Part model, mm, in its own coordinate system. Face numbers are marked on the shaded views. A direction names the side the tool comes from. Coordinates: 2 decimals unless noted, no trailing zeros. Loops run counter-clockwise (first coordinate to the right, second up) from the corner with the lowest first, then second, coordinate; pieces in that order, holes last. Notation, with made-up numbers: M -34,-31.75 L 15,-31.75 A15 ccw 15,-15.75 Z; hole C -24.75,-31.5 d1. An arc over 180 degrees is marked long. Use CSV: the item, a comma, the result in double quotes. Start each with the question number.
from build123d import *

# Parameters (mm, degrees)
SKETCH_1_R          = 15
EXTRUDE_1_DEPTH     = 35
SKETCH_2_R          = 1.4
CUT_EXTRUDE_1_DEPTH = 41.926763859
SKETCH_4_W          = 10.3
SKETCH_4_H          = 8.64
SKETCH_4_W_2        = 6.34
SKETCH_4_H_2        = 6.34
EXTRUDE_2_DEPTH     = 8
SKETCH_5_W          = 10.3
SKETCH_5_H          = 20.03
CUT_EXTRUDE_2_DEPTH = 5
CUT_EXTRUDE_3_DEPTH = 50.751390935
CUT_EXTRUDE_4_DEPTH = 37.742346142
SKETCH_8_W          = 2.3
SKETCH_8_H          = 6.34
EXTRUDE_3_DEPTH     = 1.6
SKETCH_10_W         = 2.02
SKETCH_10_H         = 3
SKETCH_11_W         = 6.34
SKETCH_11_H         = 6.34
CUT_EXTRUDE_5_DEPTH = 6.5
SKETCH_12_W         = 2.02
SKETCH_12_H         = 3
CUT_EXTRUDE_7_DEPTH = 5
SKETCH_16_R         = 3.19
CUT_EXTRUDE_8_DEPTH = 1.2
CUT_EXTRUDE_9_DEPTH = 41.926763859
CHAMFER_1_SIZE      = 1.1
CHAMFER_2_SIZE      = 1


with BuildPart() as part:
    # 草图1 → 凸台-拉伸1 (new body)
    with BuildSketch(Plane(origin=(0, 0, 0), x_dir=(1, 0, 0), z_dir=(0, 1, 0))):
        with Locations(Location((0, 0, 0), (0, 0, 270))):
            Circle(SKETCH_1_R)
    extrude(amount=EXTRUDE_1_DEPTH)

    # 草图2 → 切除-拉伸1 (cut, through all)
    with BuildSketch(Plane(origin=(0, 35, 0), x_dir=(1, 0, 0), z_dir=(0, 1, 0))):
        with Locations(Location((9, 0, 0), (0, 0, 270))):
            Circle(SKETCH_2_R)
        with Locations(Location((-9, 0, 0), (0, 0, 90))):
            Circle(SKETCH_2_R)
    extrude(amount=-CUT_EXTRUDE_1_DEPTH, mode=Mode.SUBTRACT)

    # 草图4 → 凸台-拉伸2 (add)
    with BuildSketch(Plane(origin=(0, 35, 0), x_dir=(1, 0, 0), z_dir=(0, 1, 0))):
        with Locations((0, -9.35)):
            Rectangle(SKETCH_4_W, SKETCH_4_H)
        with Locations((0, -9)):
            Rectangle(SKETCH_4_W_2, SKETCH_4_H_2, mode=Mode.SUBTRACT)
    extrude(amount=EXTRUDE_2_DEPTH)

    # 草图5 → 切除-拉伸2 (cut)
    with BuildSketch(Plane(origin=(0, 35, 0), x_dir=(1, 0, 0), z_dir=(0, 1, 0))):
        with Locations((0, 4.985)):
            Rectangle(SKETCH_5_W, SKETCH_5_H)
    extrude(amount=-CUT_EXTRUDE_2_DEPTH, mode=Mode.SUBTRACT)

    # 草图6 → 切除-拉伸3 (cut, through all)
    with BuildSketch(Plane(origin=(0, 0, 5.03), x_dir=(-1, 0, 0), z_dir=(0, 0, -1))):
        Polygon((-6.15, 32.5), (-5.15, 33.75), (-5.15, 31.25), align=None)
        Polygon((6.15, 32.5), (5.15, 33.75), (5.15, 31.25), align=None)
    extrude(amount=CUT_EXTRUDE_3_DEPTH, mode=Mode.SUBTRACT)

    # 草图7 → 切除-拉伸4 (cut, through all)
    with BuildSketch(Plane(origin=(0, 30, 0), x_dir=(1, 0, 0), z_dir=(0, 1, 0))):
        with BuildLine():
            Line((-5.15, 14.088204286), (-5.15, 4.97))
            Line((-5.15, 4.97), (5.15, 4.97))
            Line((5.15, 4.97), (5.15, 14.088204286))
            ThreePointArc((5.15, 14.088204286), (0, 15), (-5.15, 14.088204286))
        make_face()
    extrude(amount=-CUT_EXTRUDE_4_DEPTH, mode=Mode.SUBTRACT)

    # 草图8 → 凸台-拉伸3 (add)
    with BuildSketch(Plane(origin=(0, 35, 0), x_dir=(1, 0, 0), z_dir=(0, 1, 0))):
        with Locations((0, -9)):
            Rectangle(SKETCH_8_W, SKETCH_8_H)
    extrude(amount=EXTRUDE_3_DEPTH)

    # 切除-扫描1: sweep along a path in 草图9
    with BuildLine(Plane(origin=(0, 0, 0), x_dir=(0, 0, -1), z_dir=(1, 0, 0))) as sweep_1_path:
        Line((-9, 35), (-9, 27.97))
        Line((-9, 27.97), (-3.03, 22))
        Line((-3.03, 22), (4.97, 22))
    # 草图10 → 切除-扫描1 (sweep, cut)
    with BuildSketch(Plane(origin=(0, 35, 0), x_dir=(1, 0, 0), z_dir=(0, 1, 0))):
        with Locations((2.16, -9)):
            Rectangle(SKETCH_10_W, SKETCH_10_H)
        with Locations((-2.16, -9)):
            Rectangle(SKETCH_10_W, SKETCH_10_H)
    sweep(path=sweep_1_path.line, transition=Transition.RIGHT, mode=Mode.SUBTRACT)

    # 草图11 → 切除-拉伸5 (cut)
    with BuildSketch(Plane.XZ):
        with Locations((0, 9)):
            Rectangle(SKETCH_11_W, SKETCH_11_H)
    extrude(amount=-CUT_EXTRUDE_5_DEPTH, mode=Mode.SUBTRACT)

    # 切除-扫描2: sweep along a path in 草图13
    with BuildLine(Plane(origin=(0, 0, 0), x_dir=(0, 0, -1), z_dir=(1, 0, 0))) as sweep_2_path:
        Line((-9, 6.5), (-9, 13.5))
        Line((-9, 13.5), (-4.5, 18))
        Line((-4.5, 18), (4.97, 18))
    # 草图12 → 切除-扫描2 (sweep, cut)
    with BuildSketch(Plane.XZ.offset(-6.5)):
        with Locations((-2.16, 9)):
            Rectangle(SKETCH_12_W, SKETCH_12_H)
        with Locations((2.16, 9)):
            Rectangle(SKETCH_12_W, SKETCH_12_H)
    sweep(path=sweep_2_path.line, transition=Transition.RIGHT, mode=Mode.SUBTRACT)

    # 草图15 → 切除-拉伸7 (cut)
    with BuildSketch(Plane(origin=(0, 35, 0), x_dir=(1, 0, 0), z_dir=(0, 1, 0))):
        Polygon((9, 2.615396719), (6.735, 1.30769836), (6.735, -1.30769836), (9, -2.615396719), (11.265, -1.30769836), (11.265, 1.30769836), align=None)
        Polygon((-11.265, -1.30769836), (-11.265, 1.30769836), (-9, 2.615396719), (-6.735, 1.30769836), (-6.735, -1.30769836), (-9, -2.615396719), align=None)
    cut_extrude_7 = extrude(amount=-CUT_EXTRUDE_7_DEPTH, mode=Mode.SUBTRACT)

    # 草图16 → 切除-拉伸8 (cut)
    with BuildSketch(Plane(origin=(0, 35, 0), x_dir=(1, 0, 0), z_dir=(0, 1, 0))):
        with Locations(Location((9, 0, 0), (0, 0, 270))):
            Circle(SKETCH_16_R)
        with Locations(Location((-9, 0, 0), (0, 0, 90))):
            Circle(SKETCH_16_R)
    cut_extrude_8 = extrude(amount=-CUT_EXTRUDE_8_DEPTH, mode=Mode.SUBTRACT)

    # 镜向1: 切除-拉伸7, 切除-拉伸8 across plane
    add(cut_extrude_7.mirror(Plane.ZX.offset(17.5)), mode=Mode.SUBTRACT)
    add(cut_extrude_8.mirror(Plane.ZX.offset(17.5)), mode=Mode.SUBTRACT)

    # 草图17 → 切除-拉伸9 (cut, through all)
    with BuildSketch(Plane(origin=(0, 35, 0), x_dir=(1, 0, 0), z_dir=(0, 1, 0))):
        with BuildLine():
            Line((14.5, 3.840572874), (14.5, -3.840572874))
            ThreePointArc((14.5, -3.840572874), (15, 0), (14.5, 3.840572874))
        make_face()
        with BuildLine():
            Line((-14.5, 3.840572874), (-14.5, -3.840572874))
            ThreePointArc((-14.5, -3.840572874), (-15, 0), (-14.5, 3.840572874))
        make_face()
    extrude(amount=-CUT_EXTRUDE_9_DEPTH, mode=Mode.SUBTRACT)

    # 倒角1
    # the kernel refuses this chamfer: 1.1 mm, written as the material it adds along each edge
    with BuildSketch(Plane(origin=(-3.17, 19.5, 7.95017163), x_dir=(-0.027495876610586133, -0.9996219169112966, 0), z_dir=(0, 0, -1))) as chamfer_1_piece_1:
        Polygon((CHAMFER_1_SIZE * 0.999621916911, -CHAMFER_1_SIZE * 0.0274958766106), (-CHAMFER_1_SIZE * 0.0274958766106, -CHAMFER_1_SIZE * 0.999621916911), (0, 0), align=None)
    extrude(amount=12.92017163)
    with BuildSketch(Plane(origin=(-1.15, 19.5, 7.95017163), x_dir=(0.02749587661058633, -0.9996219169112966, 0), z_dir=(0, 0, -1)), Plane(origin=(3.17, 19.5, 7.95017163), x_dir=(0.027495876610586525, -0.9996219169112966, 0), z_dir=(0, 0, -1)), Plane(origin=(1.15, 19.5, 7.95017163), x_dir=(0.9996219169112966, 0.02749587661058971, 0), z_dir=(0, 0, -1))) as chamfer_1_piece_2:
        Polygon((CHAMFER_1_SIZE * 0.999621916911, CHAMFER_1_SIZE * 0.0274958766106), (-CHAMFER_1_SIZE * 0.0274958766106, CHAMFER_1_SIZE * 0.999621916911), (0, 0), align=None)
    extrude(amount=12.92017163)

    # 倒角2
    chamfer_2_edges = [part.edges().sort_by_distance(p)[0] for p in [
        (3.17, 23.5, -1.280660172),
        (1.15, 23.5, -1.280660172),
        (-1.15, 23.5, -1.280660172),
        (-3.17, 23.5, -1.280660172),
    ]]
    chamfer(chamfer_2_edges, length=CHAMFER_2_SIZE)


solid = part.part
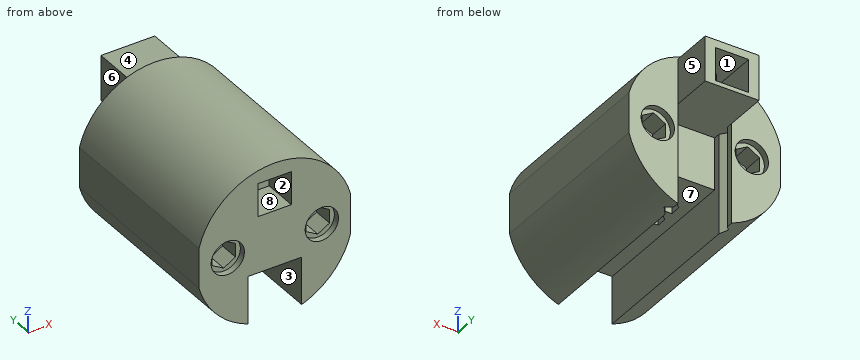
1. Slice it at C-C, the plane x = 9.5. List the corners of the cut face in (y, z), and give its area (3 significant figures).
2. Two-plate mould, pull along Z, no slides. Class the marked faces 1, 2, 3 and 4: pulls with the +Z half, pulls with the -Z half, needs draft (parallel to the pull), parting line crosses it, or undercut.
3. Slice it at A-A, the plane y = 34.5. List the corners of the cut face in (x, z), and give its area (3 significant figures).
4. Slice it at B-B, the plane z = -11.25. List the corners of the cut face in (x, y).
5. Pin check, flat tips, straight feed: pin 1 (2 mm diameter, centred on x = -2, y = 27, fed in from +Z); pin 2 (2 mm diameter, centred on y = 36.5, z = 12, fed in from -X); pin 3 (1.2 mm diameter, centred on x = 0, z = 9.5, fed in from +Y). Stop position of each tip, or through.
6. Slice it at D-D, the plane z = 0. State how many separate pieces and enclosed holes the cut face has, and give its area (3 significant figures).
7. Wall check: probe 1 along X at (y, z) = (0.7, 0); probe 2 along X at (y, z) = (16, 0); probe 3 along X at (y, z) = (34.5, 0). Give the ranges that are in metal, low to high.
8. Tool access for the marked faces 5, 6, 7 and 8: list every direction of +Z, -Z, +X, -X, +Y, -Y with a clear straight run to the whole face (end or side of a thin tool).
Found:
1,outline,"M 0,-11.61 L 35,-11.61 L 35,-3.15 L 33.8,-3.15 L 33.8,-2.33 L 30,-2.33 L 30,-1.31 L 5,-1.31 L 5,-2.33 L 1.2,-2.33 L 1.2,-3.15 L 0,-3.15 Z; M 0,3.15 L 1.2,3.15 L 1.2,2.33 L 5,2.33 L 5,1.31 L 30,1.31 L 30,2.33 L 33.8,2.33 L 33.8,3.15 L 35,3.15 L 35,11.61 L 0,11.61 Z"
1,area,"697 mm^2"
2,face 1,"undercut"
2,face 2,"undercut"
2,face 3,"needs draft"
2,face 4,"pulls with the +Z half"
3,outline,"M -14.5,-3.84 A15 ccw -5.15,-14.09 L -5.15,5.03 L 5.15,5.03 L 5.15,-14.09 A15 ccw 14.5,-3.84 L 14.5,3.84 A15 ccw -14.5,3.84 Z; hole C -9,0 d6.38; hole M -3.17,7.5 L -1.15,7.5 L -1.15,10.5 L -3.17,10.5 Z; hole M 1.15,7.5 L 3.17,7.5 L 3.17,10.5 L 1.15,10.5 Z; hole C 9,0 d6.38"
3,area,"422 mm^2"
4,outline,"M -9.92,0 L -5.15,0 L -5.15,31.25 L -6.15,32.5 L -5.15,33.75 L -5.15,35 L -9.92,35 Z; M 5.15,0 L 9.92,0 L 9.92,35 L 5.15,35 L 5.15,33.75 L 6.15,32.5 L 5.15,31.25 Z"
5,pin 1,"z = 14.97"
5,pin 2,"x = -5.15"
5,pin 3,"y = 36.6"
6,separate pieces,"3"
6,enclosed holes,"4"
6,area,"702 mm^2"
7,probe 1,"-14.5 to -12.19, -5.81 to 5.81, 12.19 to 14.5"
7,probe 2,"-14.5 to -10.4, -7.6 to 7.6, 10.4 to 14.5"
7,probe 3,"-14.5 to -12.19, -5.81 to -5.15, 5.15 to 5.81, 12.19 to 14.5"
8,face 5,"+Z, -Z, +X, +Y"
8,face 6,"+Z, -Z, -X, +Y"
8,face 7,"-Z, +Y, -Y"
8,face 8,"-Y"
